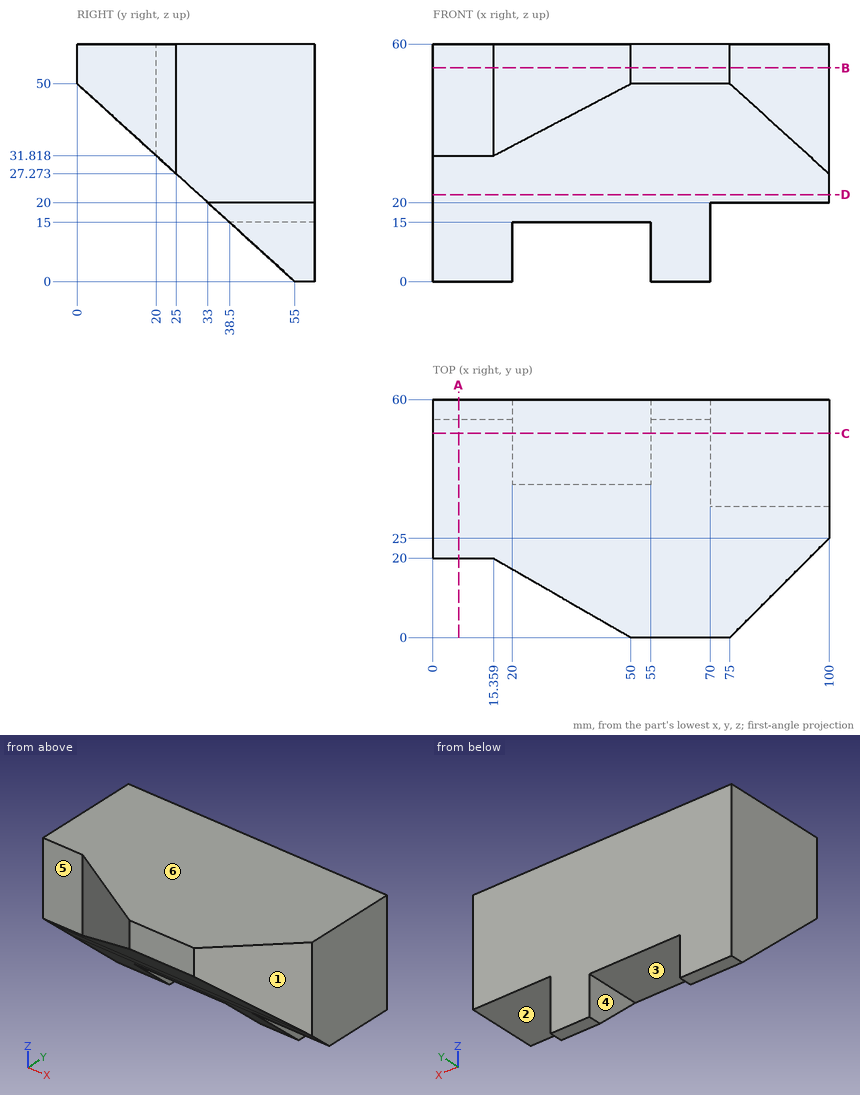
Part print with two shaded views. Sizes in mm from the minimum x, y, z corner. A direction names the side the tool comes from. Coordinates: 2 decimals unless noted, no trailing zeros. Write each loop counter-clockwise with the first axis right and the second up, starting at its lowest first coordinate (ties: lowest second). Pieces come first, ordered by that corner, then holes. Notation, with made-up numbers: (88.25, 26) - (125.25, 26) arc R13 cw to (125.25, 35) - close; hole circle Ø5 at (39, 85.5). An arc over 180 degrees is marked (long way). Put each result on its own line as item: value.
1. Band-saw the part on D-D (z = 22). Write the cut outline in (x, y).
Final values:
outline: (0, 30.8) - (100, 30.8) - (100, 60) - (0, 60) - close
2. Band-saw the part on A-A (x = 6.5). Write the cut outline in (y, z), then the cut area to 3 significant figures.
Final values:
outline: (20, 31.82) - (55, 0) - (60, 0) - (60, 60) - (20, 60) - close
area: 1,840 mm²
3. Probe line 1 along Y through (x, z) = (9, 20); line 2 along Z through (x, y) = (88, 47); line 3 along Y through (x, z) = (12, 22). List the from-to ranges inside material, lowest first. Write a range as [from, to].
Final values:
line 1: y = [33, 60]
line 2: z = [20, 60]
line 3: y = [30.8, 60]
4. Flat gauge pins, fed straight in: pin 1 Ø6 at (y, z) = (45, 9) entering from +X; pin 2 Ø2 at (x, y) = (60.5, 18.5) entering from -Z; pin 3 Ø8 at (x, y) = (88, 45.5) entering from -Z. Where does each tip first touch, or does it go through?
Final values:
pin 1: stops at x = 70
pin 2: stops at z = 32.27
pin 3: stops at z = 20
5. Band-saw the part on C-C (y = 51.5). Write the cut outline in (x, z), then the cut area to 3 significant figures.
Final values:
outline: (0, 3.18) - (20, 3.18) - (20, 15) - (55, 15) - (55, 3.18) - (70, 3.18) - (70, 20) - (100, 20) - (100, 60) - (0, 60) - close
area: 4,760 mm²
6. Band-saw the part on B-B (z = 54). Write the cut outline in (x, y), then the cut area to 3 significant figures.
Final values:
outline: (0, 20) - (15.36, 20) - (50, 0) - (75, 0) - (100, 25) - (100, 60) - (0, 60) - close
area: 5,030 mm²
7. 3-axis set-ups, long thin cutter, end or side, ignore diameter. For the marked faces 4, 5 and 6: which of +Z, -Z, +X, -X, +Y, -Y reach the whole face in a straight line?
Final values:
face 4: -Z, +Y, -Y
face 5: +Z, -Z, -X, -Y
face 6: +Z, +X, -X, +Y, -Y
8. Two-plate mould, pull along X, no slides. Class the marked faces 1, 2 and 3: +X half, -X half, draft (parallel to the pull), parting line (faces both ways), or undercut.
Final values:
face 1: +X half
face 2: draft
face 3: undercut
